Read the model definition and answer for the solid it produces. Units are mm, in the model's axes. A direction names the side the tool comes from. Give positions to 0.01 mm unless a question says otherwise; leave off trailing zeros. Order: outer loops, then holes, each group sorted by start corner. A loop starts at its lowest first (then second) coordinate and runs counter-clockwise, first axis right, second up. Notation, with made-up numbers: (-32, 29.25) -> (-14, 29.25) arc R20 cw to (-14, 58.25) -> close; hole circle Ø9 at (-38, 80). An arc over 180 degrees is marked (long way). Use one line per item in the form item = value.
```python
from build123d import *

# Parameters (mm, degrees)
SKETCH1_R           = 5.6
BOSS_EXTRUDE1_DEPTH = 4.8
SKETCH2_R           = 2.5
CUT_EXTRUDE1_DEPTH  = 4.8
SKETCH3_OUTSIDE_W   = 16.51
SKETCH3_OUTSIDE_H   = 16.51
CUT_EXTRUDE2_DEPTH  = 3
FILLET1_R           = 0.3


with BuildPart() as part:
    # Sketch1 → Boss-Extrude1 (new body)
    with BuildSketch(Plane(origin=(0, 0, 0), x_dir=(1, 0, 0), z_dir=(0, 1, 0))):
        Circle(SKETCH1_R)
    extrude(amount=BOSS_EXTRUDE1_DEPTH)

    # Sketch2 → Cut-Extrude1 (cut)
    with BuildSketch(Plane(origin=(0, 4.8, 0), x_dir=(1, 0, 0), z_dir=(0, 1, 0))):
        Circle(SKETCH2_R)
    extrude(amount=-CUT_EXTRUDE1_DEPTH, mode=Mode.SUBTRACT)

    # Sketch3 outside → Cut-Extrude2 (cut)
    with BuildSketch(Plane(origin=(0, 4.8, 0), x_dir=(1, 0, 0), z_dir=(0, 1, 0))):
        Rectangle(SKETCH3_OUTSIDE_W, SKETCH3_OUTSIDE_H)
        Polygon((4.5033321, 0), (2.25166605, 3.9), (-2.25166605, 3.9), (-4.5033321, 0), (-2.25166605, -3.9), (2.25166605, -3.9), align=None, mode=Mode.SUBTRACT)
    extrude(amount=-CUT_EXTRUDE2_DEPTH, mode=Mode.SUBTRACT)

    # Fillet1
    fillet1_edges = [part.edges().sort_by_distance(p)[0] for p in [
        (0, 1.8, 3.9),
        (3.377499075, 1.8, 1.95),
        (3.377499075, 1.8, -1.95),
        (0, 1.8, -3.9),
        (-3.377499075, 1.8, -1.95),
        (-3.377499075, 1.8, 1.95),
        (-5.6, 1.8, 0),
        (-5.6, 0, 0),
        (3.377499075, 4.8, 1.95),
        (0, 4.8, 3.9),
        (-3.377499075, 4.8, 1.95),
        (-3.377499075, 4.8, -1.95),
        (0, 4.8, -3.9),
        (3.377499075, 4.8, -1.95),
        (-2.5, 0, 0),
        (-2.5, 4.8, 0),
    ]]
    fillet(fillet1_edges, radius=FILLET1_R)


solid = part.part
```
Item 1: Given pin 1 Ø2.5 at (x, y) = (-1, 3.5) entering from -Z; pin 2 Ø2.5 at (x, y) = (0, 3.5) entering from +Z; pin 3 Ø1 at (y, z) = (3.5, 2) entering from -X, each flat-ended and moving along its own axis, determine where each tip first touches the part or whether it passes through.
Checks:
pin_1 = -3.9
pin_2 = 3.9
pin_3 = -3.64
Item 2: Which of the six approach directions +Z, -Z, +X, -X, +Y, -Y give full straight-line access (tool end or side, diameter ignored) to faces 5 (the flat face through (4, 1.8, -2)), 6 (the flat face through (3.393, 3.317, -1.923)), 7 (the flat face through (-3.36, 3.32, -1.98)), 8 (the flat face through (0, 3, 3.9))?
Checks:
face_5 = +Y
face_6 = -Z, +X, +Y
face_7 = -Z, -X, +Y
face_8 = +Z, +X, -X, +Y
Item 3: The part is cut by section C-C on y = 1.15. Give the vertices of the cut face in (x, z).
Checks:
outline = circle Ø11.2 at (0, 0); hole circle Ø5 at (0, 0)
Item 4: Straight lines are drawn through the part: L1, parallel to Z at x = 0, y = 2.15; L2, parallel to Z at x = 0, y = 1.3; L3, parallel to Y at x = -3.5, z = 4. For each, find the intervals that lie inside material, in ascending order. Write a range as from..to.
Checks:
L1 = -3.9..-2.5, 2.5..3.9
L2 = -5.6..-2.5, 2.5..5.6
L3 = 0..1.8
Item 5: Determine the mould class of faces 1 (the flat face through (-3.393, 3.317, 1.923)), 2 (the cylindrical face through (-0.54, 2.43, 2.44)), 3 (the cylindrical face through (3.473, 1.886, 1.966)), 4 (the flat face through (1, 4.8, -3)) for opening direction X: +X half, -X half, draft (parallel to the pull), parting line (faces both ways), or undercut.
Checks:
face_1 = -X half
face_2 = undercut
face_3 = +X half
face_4 = draft
Item 6: The part is cut by section B-B on y = 3.5. Give the vertices of the cut face in (x, z).
Checks:
outline = (-4.5, 0) -> (-2.25, -3.9) -> (2.25, -3.9) -> (4.5, 0) -> (2.25, 3.9) -> (-2.25, 3.9) -> close; hole circle Ø5 at (0, 0)
Item 7: The part is cut by section A-A on x = 0. Give the vertices of the cut face in (y, z).
Checks:
outline = (0, -5.3) arc R0.3 ccw to (0.3, -5.6) -> (1.5, -5.6) arc R0.3 ccw to (1.8, -5.3) -> (1.8, -4.2) arc R0.3 cw to (2.1, -3.9) -> (4.5, -3.9) arc R0.3 ccw to (4.8, -3.6) -> (4.8, -2.8) arc R0.3 ccw to (4.5, -2.5) -> (0.3, -2.5) arc R0.3 ccw to (0, -2.8) -> close; (0, 2.8) arc R0.3 ccw to (0.3, 2.5) -> (4.5, 2.5) arc R0.3 ccw to (4.8, 2.8) -> (4.8, 3.6) arc R0.3 ccw to (4.5, 3.9) -> (2.1, 3.9) arc R0.3 cw to (1.8, 4.2) -> (1.8, 5.3) arc R0.3 ccw to (1.5, 5.6) -> (0.3, 5.6) arc R0.3 ccw to (0, 5.3) -> close
